Geometry check sheet. Reference: the model listing, model coordinates, mm. A direction names the side the tool comes from. Coordinates: 2 decimals unless noted, no trailing zeros. Order: outer loops, then holes, each group sorted by start corner. A loop starts at its lowest first (then second) coordinate and runs counter-clockwise, first axis right, second up. Notation, with made-up numbers: (29.5, 61.25) - (67.5, 61.25) arc R13 cw to (67.5, 73.25) - close; hole circle Ø2 at (-32, 59.5). An arc over 180 degrees is marked (long way). Put each result on its own line as item: value.
from build123d import *

# Parameters (mm, degrees)
RESSALTO_EXTRUS_O1_DEPTH = 30
ESBO_O3_W                = 4.5
ESBO_O3_H                = 18
CORTE_EXTRUS_O2_DEPTH    = 28.5
RESSALTO_EXTRUS_O2_DEPTH = 2
ESBO_O5_R                = 0.5
CORTE_EXTRUS_O3_DEPTH    = 10
ESBO_O6_R                = 1
CORTE_EXTRUS_O4_DEPTH    = 10
RESSALTO_EXTRUS_O3_DEPTH = 27
RESSALTO_EXTRUS_O4_DEPTH = 5
FILETE1_R                = 15
ESBO_O11_R               = 2.6
CORTE_EXTRUS_O5_DEPTH    = 1.5
ESBO_O12_R               = 0.6
CORTE_EXTRUS_O6_DEPTH    = 4.5
CHANFRO1_SIZE            = 0.5


with BuildPart() as part:
    # Esboço1 → Ressalto-extrusão1 (new body)
    with BuildSketch(Plane.XY):
        Polygon((-32.5, 31.319481807), (32.5, 31.319481807), (28.25, -13.680518193), (20.25, -13.680518193), (20.25, 8.319481807), (-20.25, 8.319481807), (-20.25, -13.680518193), (-28.25, -13.680518193), align=None)
    extrude(amount=RESSALTO_EXTRUS_O1_DEPTH)

    # Esboço3 → Corte-extrusão2 (cut)
    with BuildSketch(Plane(origin=(40, 0, 0), x_dir=(0, 0, -1), z_dir=(1, 0, 0))):
        with Locations((-7.75, -4.680518193)):
            Rectangle(ESBO_O3_W, ESBO_O3_H)
    extrude(amount=-CORTE_EXTRUS_O2_DEPTH, mode=Mode.SUBTRACT)

    # Esboço4 → Ressalto-extrusão2 (add)
    with BuildSketch(Plane(origin=(0, 0, 0), x_dir=(-1, 0, 0), z_dir=(0, 0, -1))):
        Polygon((-32.5, 31.319481807), (32.5, 31.319481807), (28.25, -13.680518193), (20.25, -13.680518193), (-20.25, -13.680518193), (-28.25, -13.680518193), align=None)
    extrude(amount=RESSALTO_EXTRUS_O2_DEPTH)

    # Esboço5 → Corte-extrusão3 (cut)
    with BuildSketch(Plane.XY.offset(30)):
        with Locations((-24, 3.019481807)):
            Circle(ESBO_O5_R)
        with Locations((24, 3.019481807)):
            Circle(ESBO_O5_R)
        with Locations((-24, -6.980518193)):
            Circle(ESBO_O5_R)
        with Locations((24, -6.980518193)):
            Circle(ESBO_O5_R)
    extrude(amount=-CORTE_EXTRUS_O3_DEPTH, mode=Mode.SUBTRACT)

    # Esboço6 → Corte-extrusão4 (cut)
    with BuildSketch(Plane(origin=(0, 31.319481807, 0), x_dir=(1, 0, 0), z_dir=(0, 1, 0))):
        with Locations((-25.5, -5)):
            Circle(ESBO_O6_R)
        with Locations((-25.5, -23)):
            Circle(ESBO_O6_R)
        with Locations((25.5, -5)):
            Circle(ESBO_O6_R)
        with Locations((25.5, -23)):
            Circle(ESBO_O6_R)
    extrude(amount=-CORTE_EXTRUS_O4_DEPTH, mode=Mode.SUBTRACT)

    # Esboço7 → Ressalto-extrusão3 (add)
    with BuildSketch(Plane.XY.offset(30)):
        Polygon((-32.5, 31.319481807), (32.5, 31.319481807), (31.933333333, 25.319481807), (-31.933333333, 25.319481807), align=None)
    extrude(amount=RESSALTO_EXTRUS_O3_DEPTH)

    # Esboço10 → Ressalto-extrusão4 (add)
    with BuildSketch(Plane(origin=(20, 0, 0), x_dir=(0, 0, -1), z_dir=(1, 0, 0))):
        Polygon((-30, 25.319481807), (-30, 10.319481807), (-52, 25.319481807), align=None)
    ressalto_extrus_o4 = extrude(amount=RESSALTO_EXTRUS_O4_DEPTH)

    # Espelhar1: Ressalto-extrusão4 across plane
    add(ressalto_extrus_o4.mirror(Plane(origin=(0, 0, 0), x_dir=(0, 0, 1), z_dir=(1, 0, 0))))

    # Filete1
    filete1_edges = [part.edges().sort_by_distance(p)[0] for p in [
        (-32.216666667, 28.319481807, 57),
        (32.216666667, 28.319481807, 57),
    ]]
    fillet(filete1_edges, radius=FILETE1_R)

    # Esboço11 → Corte-extrusão5 (cut)
    with BuildSketch(Plane(origin=(0, 31.319481807, 0), x_dir=(1, 0, 0), z_dir=(0, 1, 0))):
        with Locations((0, -50.55)):
            Circle(ESBO_O11_R)
    extrude(amount=-CORTE_EXTRUS_O5_DEPTH, mode=Mode.SUBTRACT)

    # Esboço12 → Corte-extrusão6 (cut)
    with BuildSketch(Plane(origin=(0, 29.819481807, 0), x_dir=(1, 0, 0), z_dir=(0, 1, 0))):
        with Locations((0, -50.55)):
            Circle(ESBO_O12_R)
    extrude(amount=-CORTE_EXTRUS_O6_DEPTH, mode=Mode.SUBTRACT)

    # Chanfro1
    chanfro1_edges = [part.edges().sort_by_distance(p)[0] for p in [
        (-0.6, 25.319481807, 50.55),
    ]]
    chamfer(chanfro1_edges, length=CHANFRO1_SIZE)


solid = part.part
Q1. Draft check along Z on faces 6 (the flat face through (-1, 29.819, 51)), 7 (the flat face through (0, 10, 30)), 8 (the flat face through (-25, 20, 38)). Enter one of: pulls with the +Z half, pulls with the -Z half, needs draft (parallel to the pull), parting line crosses it, or undercut.
Answer block:
face 6: undercut
face 7: pulls with the +Z half
face 8: needs draft
Q2. Section check B-B on z = 9. Record the boundary of the cut face in (x, y), then the cut area to 3 significant figures.
Answer block:
outline: (-32.5, 31.32) - (-28.25, -13.68) - (-20.25, -13.68) - (-20.25, 8.32) - (20.25, 8.32) - (20.25, 4.32) - (29.95, 4.32) - (32.5, 31.32) - close
area: 1,680 mm^2
Q3. Thickness scan on L1, parallel to Y at x = -24, z = 27.25; L2, parallel to Z at x = 0, y = 30.3; L3, parallel to Z at x = -6.5, y = 14. Record the ranges inside material, lowest first. Write a range as [from, to].
Answer block:
L1: y = [-13.68, -7.48], [-6.48, 2.52], [3.52, 31.32]
L2: z = [-2, 47.95], [53.15, 57]
L3: z = [-2, 30]
Q4. Depth check by flat-ended pin: pin 1 Ø16.5 at (y, z) = (14.5, 38) entering from +X; pin 2 Ø4 at (y, z) = (15.5, 35.5) entering from -X; pin 3 Ø0.8 at (x, y) = (-24, -7) entering from +Z. Enter the tip coordinate at first touch or a pass-through.
Answer block:
pin 1: stops at x = 31.1
pin 2: stops at x = -25
pin 3: stops at z = 20
Q5. Section check A-A on x = 9.5. Record the boundary of the cut face in (y, z), then the cut area to 3 significant figures.
Answer block:
outline: (-13.68, -2) - (31.32, -2) - (31.32, 57) - (25.32, 57) - (25.32, 30) - (8.32, 30) - (8.32, 0) - (-13.68, 0) - close
area: 942 mm^2
Q6. Access from +Z, -Z, +X, -X, +Y, -Y to the whole of each face (thin tool, end or side, straight path). Record for faces 1 (the flat face through (-20, 20, 38)), 2 (the flat face through (25, 20, 38)), 3 (the flat face through (24, -13.681, 20)), 4 (the flat face through (25, 21.319, 5)), 5 (the flat face through (25, 4.319, 8)).
Answer block:
face 1: +Z, -Y
face 2: +Z, +X, -Y
face 3: +Z, -Z, +X, -X, -Y
face 4: +Y
face 5: +X, -Y
Q7. Section check C-C on z = 35. Record the boundary of the cut face in (x, y).
Answer block:
outline: (-32.5, 31.32) - (-31.93, 25.32) - (-25, 25.32) - (-25, 13.73) - (-20, 13.73) - (-20, 25.32) - (20, 25.32) - (20, 13.73) - (25, 13.73) - (25, 25.32) - (31.93, 25.32) - (32.5, 31.32) - close
